```python
from build123d import *

# Parameters (mm, degrees)
SKETCH_370_W           = 89
SKETCH_370_H           = 60
EXTRUDE_438_DEPTH      = 2
CUT_EXTRUDE_684_DEPTH  = 2
SKETCH_734_W           = 2
SKETCH_734_H           = 25
CUT_EXTRUDE_885_DEPTH  = 2
SKETCH_933_W           = 8
SKETCH_933_H           = 2
EXTRUDE_1139_DEPTH     = 2
SKETCH_1188_W          = 8
SKETCH_1188_H          = 2
EXTRUDE_1389_DEPTH     = 2
SKETCH_1437_W          = 8
SKETCH_1437_H          = 2
EXTRUDE_1598_DEPTH     = 2
CUT_EXTRUDE_2168_DEPTH = 1
SKETCH_2222_R          = 2
CUT_EXTRUDE_2716_DEPTH = 3


with BuildPart() as part:
    # Sketch 370 → Extrude 438 (new body)
    with BuildSketch(Plane(origin=(0, 0, 0), x_dir=(1, 0, 0), z_dir=(0, 1, 0))):
        Rectangle(SKETCH_370_W, SKETCH_370_H)
    extrude(amount=EXTRUDE_438_DEPTH)

    # Sketch 488 → Cut-Extrude 684 (cut)
    with BuildSketch(Plane(origin=(0, 2, 0), x_dir=(1, 0, 0), z_dir=(0, 1, 0))):
        Polygon((-44.5, -30), (-42.5, -30), (-42.5, 28), (9.5, 28), (9.5, 30), (-44.5, 30), align=None)
    extrude(amount=-CUT_EXTRUDE_684_DEPTH, mode=Mode.SUBTRACT)

    # Sketch 734 → Cut-Extrude 885 (cut)
    with BuildSketch(Plane(origin=(0, 2, 0), x_dir=(1, 0, 0), z_dir=(0, 1, 0))):
        with Locations((43.5, -17.5)):
            Rectangle(SKETCH_734_W, SKETCH_734_H)
    extrude(amount=-CUT_EXTRUDE_885_DEPTH, mode=Mode.SUBTRACT)

    # Sketch 933 → Extrude 1139 (add)
    with BuildSketch(Plane.ZY.offset(42.5)):
        with Locations((17, 1)):
            Rectangle(SKETCH_933_W, SKETCH_933_H)
        with Locations((0, 1)):
            Rectangle(SKETCH_933_W, SKETCH_933_H)
        with Locations((-17, 1)):
            Rectangle(SKETCH_933_W, SKETCH_933_H)
    extrude(amount=EXTRUDE_1139_DEPTH)

    # Sketch 1188 → Extrude 1389 (add)
    with BuildSketch(Plane(origin=(0, 0, -28), x_dir=(-1, 0, 0), z_dir=(0, 0, -1))):
        with Locations((31.5, 1)):
            Rectangle(SKETCH_1188_W, SKETCH_1188_H)
        with Locations((14.5, 1)):
            Rectangle(SKETCH_1188_W, SKETCH_1188_H)
        with Locations((-2.5, 1)):
            Rectangle(SKETCH_1188_W, SKETCH_1188_H)
    extrude(amount=EXTRUDE_1389_DEPTH)

    # Sketch 1437 → Extrude 1598 (add)
    with BuildSketch(Plane(origin=(42.5, 0, 0), x_dir=(0, 0, -1), z_dir=(1, 0, 0))):
        with Locations((-17, 1)):
            Rectangle(SKETCH_1437_W, SKETCH_1437_H)
    extrude(amount=EXTRUDE_1598_DEPTH)

    # Sketch 1650 → Cut-Extrude 2168 (cut)
    with BuildSketch(Plane.XZ):
        Polygon((44.5, -30), (9.5, -30), (9.5, -23), (37.5, 5), (44.5, 5), align=None)
    extrude(amount=-CUT_EXTRUDE_2168_DEPTH, mode=Mode.SUBTRACT)

    # Sketch 2222 → Cut-Extrude 2716 (cut, through all)
    with BuildSketch(Plane(origin=(0, 2, 0), x_dir=(1, 0, 0), z_dir=(0, 1, 0))):
        with Locations((13.5, -10)):
            Circle(SKETCH_2222_R)
    extrude(amount=-CUT_EXTRUDE_2716_DEPTH, mode=Mode.SUBTRACT)


solid = part.part
```
Geometry: final body of the model. Coordinates: model frame, mm. A direction names the side the tool comes from. Round coordinates to 2 decimals unless told otherwise and drop trailing zeros. Loops run counter-clockwise (first coordinate to the right, second up) from the corner with the lowest first, then second, coordinate; pieces in that order, holes last. Notation, with made-up numbers: (14.25, 35.5) -> (50.25, 35.5) arc R18 ccw to (50.25, 55.5) -> close; hole circle Ø2 at (-26, 29.25). An arc over 180 degrees is marked (long way). Use one line per item in the form item = value.
Item 1: Draft query along X for faces 1 (the flat face through (-1, 2, 0)), 2 (the flat face through (6.5, 1, -29)), 3 (the flat face through (-44.5, 1, -17)). Return one class per face: released by +X, released by -X, zero draft, split by the parting line, or undercut.
Evaluation:
face_1 = zero draft
face_2 = undercut
face_3 = released by -X
Item 2: Cut plane B-B on x = 13.5. Output: boundary loops of the cut face in (y, z).
Evaluation:
outline = (0, -19) -> (1, -19) -> (1, -30) -> (2, -30) -> (2, 8) -> (0, 8) -> close; (0, 12) -> (2, 12) -> (2, 30) -> (0, 30) -> close
Item 3: Material intervals for probe 1 along X at (y, z) = (0.55, 10); probe 2 along Z at (x, y) = (13.5, 1.45); probe 3 along Y at (x, z) = (23, -18), sorted ascending.
Evaluation:
probe_1 = -42.5 to 11.5, 15.5 to 42.5
probe_2 = -30 to 8, 12 to 30
probe_3 = 1 to 2
Item 4: Access query for faces 4 (the flat face through (-1.5, 1, -29)), 5 (the flat face through (-43, 1, 13)), 6 (the flat face through (42.5, 1, 26)), 7 (the flat face through (-43, 1, -21)). Directions: +Z, -Z, +X, -X, +Y, -Y. A direction counts if a zero-diameter tool reaches every point of the face in a straight line with its end or side. Return the directions, or none.
Evaluation:
face_4 = -Z, +Y, -Y
face_5 = -X, +Y, -Y
face_6 = +Z, +X, +Y, -Y
face_7 = -Z, -X, +Y, -Y
Item 5: Contact query for flat-ended pins moving along their axis: pin 1 Ø0.6 at (x, y) = (-43.5, 1.5) entering from +Z; pin 2 Ø0.6 at (x, y) = (-40.5, 0.5) entering from -Z; pin 3 Ø0.8 at (y, z) = (0.5, -25.5) entering from +X. Output: stop coordinate, or through.
Evaluation:
pin_1 = 21
pin_2 = -28
pin_3 = 9.5
Item 6: Cut plane C-C on z = -22. Output: boundary loops of the cut face in (x, y).
Evaluation:
outline = (-42.5, 0) -> (10.5, 0) -> (10.5, 1) -> (44.5, 1) -> (44.5, 2) -> (-42.5, 2) -> close
Item 7: Cut plane A-A on z = 10. Output: boundary loops of the cut face in (x, y).
Evaluation:
outline = (-42.5, 0) -> (11.5, 0) -> (11.5, 2) -> (-42.5, 2) -> close; (15.5, 0) -> (42.5, 0) -> (42.5, 2) -> (15.5, 2) -> close
